Part print with two shaded views. Sizes in mm from the minimum x, y, z corner. Round coordinates to 2 decimals unless told otherwise and drop trailing zeros. Loops run counter-clockwise (first coordinate to the right, second up) from the corner with the lowest first, then second, coordinate; pieces in that order, holes last.
(1) Cut at B-B on y = 0.7. List the corners of the cut face in (x, z) (1 decimal).
(2) Probe probe 1 along Z at (x, y) = (82, 0.85); probe 2 along X at (y, z) = (0.7, 31); probe 3 along Z at (x, y) = (56, 2.85). List the from-to ranges inside material, lowest first.
(3) Cut at C-C on z = 32. List the corners of the cut face in (x, y).
(4) Cut at A-A on x = 81.5. List the corners of the cut face in (y, z), then the cut area to 3 significant figures.
(5) Flat gauge pins, fed straight in: pin 1 (0.6 mm diameter, centred on y = 2, z = 60, fed in from +X); pin 2 (1 mm diameter, centred on y = 1, z = 1, fed in from -X); pin 3 (1.5 mm diameter, centred on x = 12.5, y = 1, fed in from -Z). Where does each tip first touch, or does it go through?
(6) Cut at D-D on x = 36. List the corners of the cut face in (y, z).
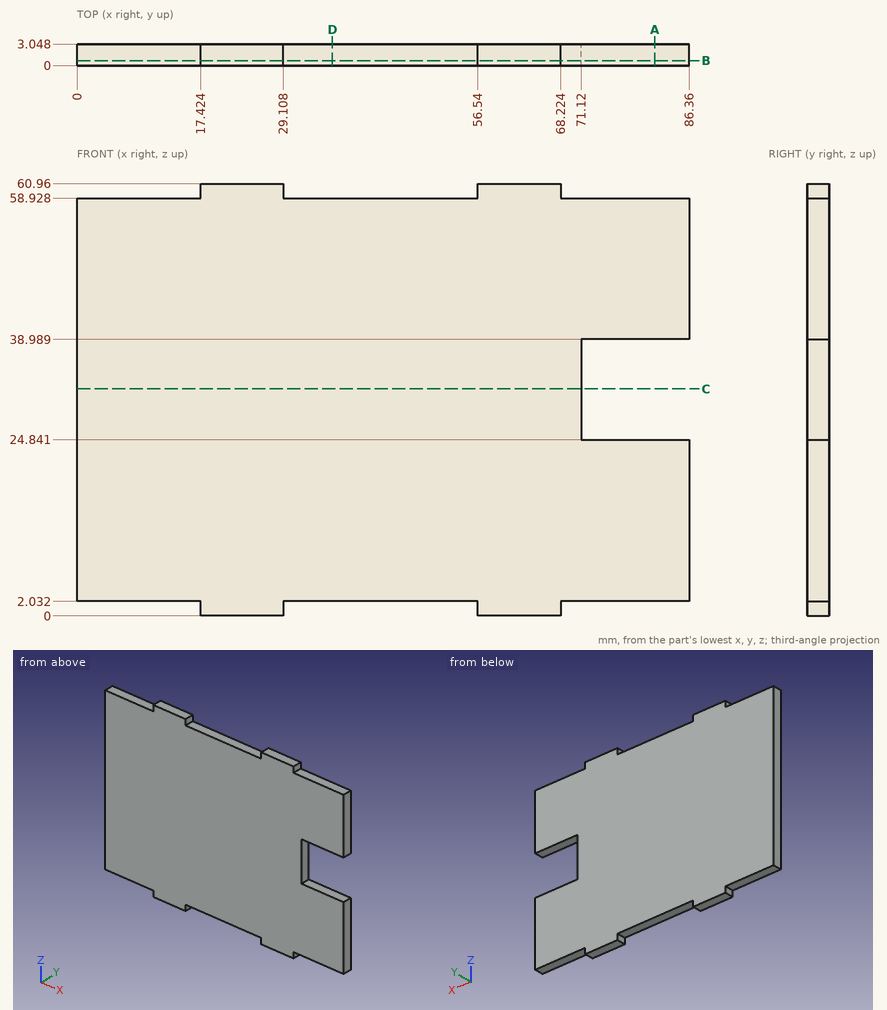
Final values:
1. outline: (0, 2) - (17.4, 2) - (17.4, 0) - (29.1, 0) - (29.1, 2) - (56.5, 2) - (56.5, 0) - (68.2, 0) - (68.2, 2) - (86.4, 2) - (86.4, 24.8) - (71.1, 24.8) - (71.1, 39) - (86.4, 39) - (86.4, 58.9) - (68.2, 58.9) - (68.2, 61) - (56.5, 61) - (56.5, 58.9) - (29.1, 58.9) - (29.1, 61) - (17.4, 61) - (17.4, 58.9) - (0, 58.9) - close
2. probe 1: z = 2.03 to 24.84, 38.99 to 58.93
2. probe 2: x = 0 to 71.12
2. probe 3: z = 2.03 to 58.93
3. outline: (0, 0) - (71.12, 0) - (71.12, 3.05) - (0, 3.05) - close
4. outline: (0, 2.03) - (3.05, 2.03) - (3.05, 24.84) - (0, 24.84) - close; (0, 38.99) - (3.05, 38.99) - (3.05, 58.93) - (0, 58.93) - close
4. area: 130 mm2
5. pin 1: stops at x = 68.22
5. pin 2: stops at x = 17.42
5. pin 3: stops at z = 2.03
6. outline: (0, 2.03) - (3.05, 2.03) - (3.05, 58.93) - (0, 58.93) - close
